Geometry check sheet. Reference: drawing and pictorial views, mm from the part's lowest x, y, z. A direction names the side the tool comes from. Coordinates: 2 decimals unless noted, no trailing zeros. Write each loop counter-clockwise with the first axis right and the second up, starting at its lowest first coordinate (ties: lowest second). Pieces come first, ordered by that corner, then holes. Notation, with made-up numbers: (-6.75, 57) -> (7.25, 57) arc R19 cw to (7.25, 80) -> close; hole circle Ø6 at (-8.5, 77). An arc over 180 degrees is marked (long way). Use a Markdown table: item, result. Add a question column.
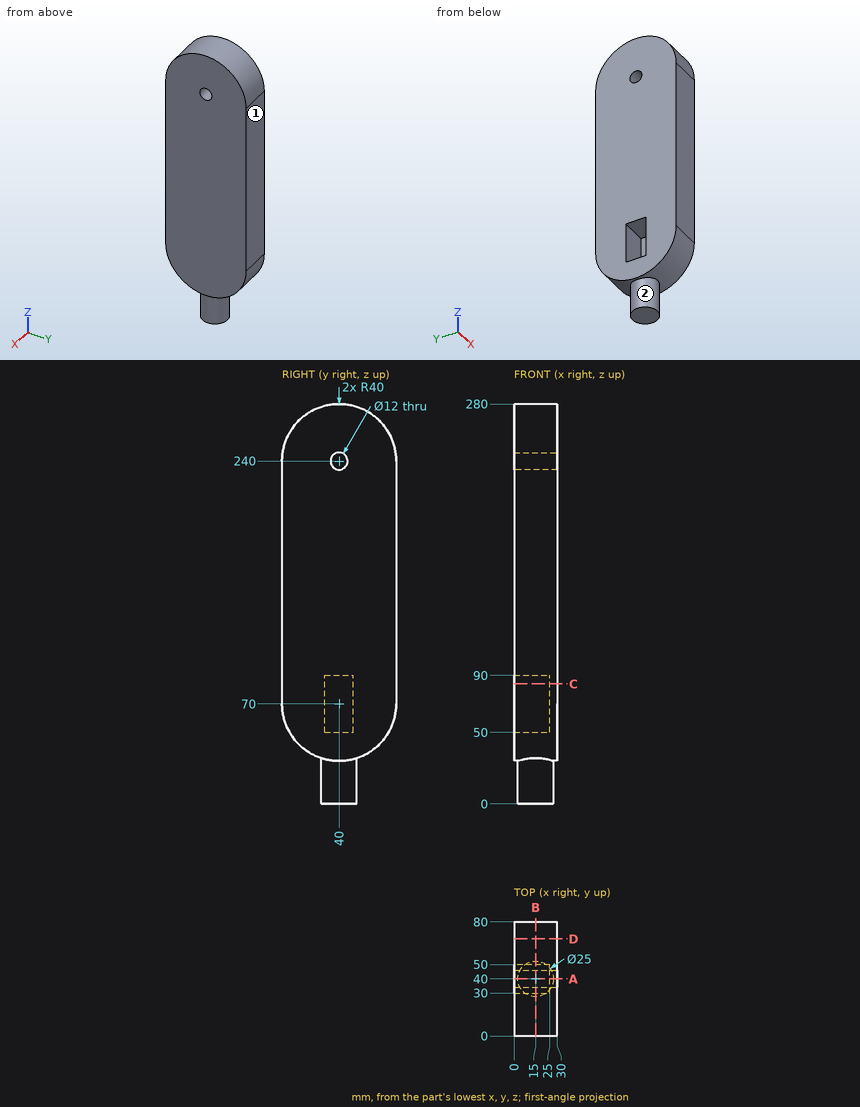
1) Cross-section at B-B on x = 15. Record the boundary of the cut face in (y, z).
2) Cross-section at D-D on y = 68. Record the boundary of the cut face in (x, z).
3) Cross-section at A-A on y = 40. Record the boundary of the cut face in (x, z), then the cut area to 3 significant figures.
4) Thickness scan on L1, parallel to Y at x = 23, z = 78; L2, parallel to Z at x = 1.5, y = 43; L3, parallel to Y at x = 20.5, z = 236.5. Record the ranges inside material, lowest first.
5) Gauge pin test, flat ends, axial feed: pin 1 (1 mm diameter, centred on x = 9.5, y = 26.5, fed in from -Z); pin 2 (12 mm diameter, centred on x = 20, z = 39.5, fed in from +Y); pin 3 (6 mm diameter, centred on x = 10.5, z = 246.5, fed in from -Y). Record the tip position at first contact, or that the pin passes through.
6) Cross-section at C-C on z = 84. Record the boundary of the cut face in (x, y).
7) Set-up check for the marked faces 1 and 2: record each of +Z, -Z, +X, -X, +Y, -Y from which the full face is reachable in a straight line by a thin tool's end or side.
Returned:
| question | item | result |
|---|---|---|
| 1 | outline | (0, 70) arc R40 ccw to (27.5, 32) -> (27.5, 0) -> (52.5, 0) -> (52.5, 32) arc R40 ccw to (80, 70) -> (80, 240) arc R40 ccw to (0, 240) -> close; hole (30, 50) -> (50, 50) -> (50, 90) -> (30, 90) -> close; hole circle Ø12 at (40, 240) |
| 2 | outline | (0, 41.43) -> (30, 41.43) -> (30, 268.57) -> (0, 268.57) -> close |
| 3 | outline | (0, 30) -> (2.5, 30) -> (2.5, 0) -> (27.5, 0) -> (27.5, 30) -> (30, 30) -> (30, 234) -> (0, 234) -> (0, 90) -> (25, 90) -> (25, 50) -> (0, 50) -> close; (0, 246) -> (30, 246) -> (30, 280) -> (0, 280) -> close |
| 3 | area | 6,890 mm² |
| 4 | L1 | y = 0 to 30, 50 to 80 |
| 4 | L2 | z = 30.11 to 50, 90 to 234.8, 245.2 to 279.89 |
| 4 | L3 | y = 0 to 35.13, 44.87 to 80 |
| 5 | pin 1 | stops at z = 32.17 |
| 5 | pin 2 | stops at y = 71.62 |
| 5 | pin 3 | stops at y = 0.15 |
| 6 | outline | (0, 0) -> (30, 0) -> (30, 80) -> (0, 80) -> (0, 50) -> (25, 50) -> (25, 30) -> (0, 30) -> close |
| 7 | face 1 | +Z, -Z, +X, -X, +Y |
| 7 | face 2 | -Z |
